```python
from build123d import *

# Parameters (mm, degrees)
SKETCH1_W            = 40
SKETCH1_H            = 40
BOSS_EXTRUDE3_DEPTH  = 2
BOSS_EXTRUDE4_DEPTH  = 6
BOSS_EXTRUDE5_DEPTH  = 2
BOSS_EXTRUDE6_START  = -6
BOSS_EXTRUDE6_DEPTH  = 6
BOSS_EXTRUDE7_DEPTH  = 2
SKETCH7_R            = 1
CUT_EXTRUDE1_DEPTH   = 5
CUT_EXTRUDE2_DEPTH   = 34
BOSS_EXTRUDE8_DEPTH  = 8
BOSS_EXTRUDE9_DEPTH  = 40
SKETCH11_W           = 40
SKETCH11_H           = 40
BOSS_EXTRUDE10_DEPTH = 2
SKETCH13_R           = 1
CUT_EXTRUDE3_DEPTH   = 5
CIRPATTERN1_COUNT    = 4


with BuildPart() as part:
    # Sketch1 → Boss-Extrude3 (new body)
    with BuildSketch(Plane(origin=(0, 0, 0), x_dir=(1, 0, 0), z_dir=(0, 1, 0))):
        Rectangle(SKETCH1_W, SKETCH1_H)
    extrude(amount=BOSS_EXTRUDE3_DEPTH)

    # Sketch5 → Boss-Extrude4 (add)
    with BuildSketch(Plane(origin=(0, 2, 0), x_dir=(1, 0, 0), z_dir=(0, 1, 0))):
        Polygon((18, -10.5), (-18, -10.5), (-18, -12.5), (20, -12.5), (20, 12.5), (-18, 12.5), (-18, 10.5), (18, 10.5), align=None)
    extrude(amount=BOSS_EXTRUDE4_DEPTH)

    # Sketch6 → Boss-Extrude5 (add)
    with BuildSketch(Plane(origin=(0, 8, 0), x_dir=(1, 0, 0), z_dir=(0, 1, 0))):
        with BuildLine():
            ThreePointArc((14, -10.5), (12, -9.5), (10, -10.5))
            Line((10, -10.5), (-10, -10.5))
            ThreePointArc((-10, -10.5), (-12, -9.5), (-14, -10.5))
            Line((-14, -10.5), (-18, -10.5))
            Line((-18, -10.5), (-18, -12.5))
            Line((-18, -12.5), (-14.449489743, -12.5))
            ThreePointArc((-14.449489743, -12.5), (-12, -14.5), (-9.550510257, -12.5))
            Line((-9.550510257, -12.5), (9.550510257, -12.5))
            ThreePointArc((9.550510257, -12.5), (12, -14.5), (14.449489743, -12.5))
            Line((14.449489743, -12.5), (20, -12.5))
            Line((20, -12.5), (20, 12.5))
            Line((20, 12.5), (14.449489743, 12.5))
            ThreePointArc((14.449489743, 12.5), (12, 14.5), (9.550510257, 12.5))
            Line((9.550510257, 12.5), (-9.550510257, 12.5))
            ThreePointArc((-9.550510257, 12.5), (-12, 14.5), (-14.449489743, 12.5))
            Line((-14.449489743, 12.5), (-18, 12.5))
            Line((-18, 12.5), (-18, 10.5))
            Line((-18, 10.5), (-14, 10.5))
            ThreePointArc((-14, 10.5), (-12, 9.5), (-10, 10.5))
            Line((-10, 10.5), (10, 10.5))
            ThreePointArc((10, 10.5), (12, 9.5), (14, 10.5))
            Line((14, 10.5), (18, 10.5))
            Line((18, 10.5), (18, -10.5))
            Line((18, -10.5), (14, -10.5))
        make_face()
    extrude(amount=BOSS_EXTRUDE5_DEPTH)

    # Sketch6<3> → Boss-Extrude6 (add)
    with BuildSketch(Plane(origin=(0, 8, 0), x_dir=(1, 0, 0), z_dir=(0, 1, 0)).offset(BOSS_EXTRUDE6_START)):
        with BuildLine():
            ThreePointArc((-9.550510257, 12.5), (-12, 14.5), (-14.449489743, 12.5))
            Line((-14.449489743, 12.5), (-9.550510257, 12.5))
        make_face()
        with BuildLine():
            ThreePointArc((14.449489743, 12.5), (12, 14.5), (9.550510257, 12.5))
            Line((9.550510257, 12.5), (14.449489743, 12.5))
        make_face()
        with BuildLine():
            Line((-9.550510257, -12.5), (-14.449489743, -12.5))
            ThreePointArc((-14.449489743, -12.5), (-12, -14.5), (-9.550510257, -12.5))
        make_face()
        with BuildLine():
            ThreePointArc((9.550510257, -12.5), (12, -14.5), (14.449489743, -12.5))
            Line((14.449489743, -12.5), (9.550510257, -12.5))
        make_face()
    extrude(amount=BOSS_EXTRUDE6_DEPTH)

    # Sketch6<4> → Boss-Extrude7 (add)
    with BuildSketch(Plane(origin=(0, 8, 0), x_dir=(1, 0, 0), z_dir=(0, 1, 0))):
        with BuildLine():
            Line((-15.5, -8), (-18, -8))
            Line((-18, -8), (-18, -10.5))
            Line((-18, -10.5), (-14, -10.5))
            ThreePointArc((-14, -10.5), (-13.118033989, -9.763932023), (-12, -9.5))
            Line((-12, -9.5), (-12, -8))
            Line((-12, -8), (-15.5, -8))
        make_face()
        with BuildLine():
            Line((12, -8), (-12, -8))
            Line((-12, -8), (-12, -9.5))
            ThreePointArc((-12, -9.5), (-10.881966011, -9.763932023), (-10, -10.5))
            Line((-10, -10.5), (10, -10.5))
            ThreePointArc((10, -10.5), (10.881966011, -9.763932023), (12, -9.5))
            Line((12, -9.5), (12, -8))
        make_face()
        with BuildLine():
            Line((12, 9.5), (12, 8))
            Line((12, 8), (15.5, 8))
            Line((15.5, 8), (15.5, -8))
            Line((15.5, -8), (12, -8))
            Line((12, -8), (12, -9.5))
            ThreePointArc((12, -9.5), (13.118033989, -9.763932023), (14, -10.5))
            Line((14, -10.5), (18, -10.5))
            Line((18, -10.5), (18, 10.5))
            Line((18, 10.5), (14, 10.5))
            ThreePointArc((14, 10.5), (13.118033989, 9.763932023), (12, 9.5))
        make_face()
        with BuildLine():
            ThreePointArc((-10, 10.5), (-10.881966011, 9.763932023), (-12, 9.5))
            Line((-12, 9.5), (-12, 8))
            Line((-12, 8), (12, 8))
            Line((12, 8), (12, 9.5))
            ThreePointArc((12, 9.5), (10.881966011, 9.763932023), (10, 10.5))
            Line((10, 10.5), (-10, 10.5))
        make_face()
        with BuildLine():
            Line((-14, 10.5), (-18, 10.5))
            Line((-18, 10.5), (-18, 8))
            Line((-18, 8), (-15.5, 8))
            Line((-15.5, 8), (-12, 8))
            Line((-12, 8), (-12, 9.5))
            ThreePointArc((-12, 9.5), (-13.118033989, 9.763932023), (-14, 10.5))
        make_face()
    extrude(amount=BOSS_EXTRUDE7_DEPTH)

    # Sketch7 → Cut-Extrude1 (cut)
    with BuildSketch(Plane(origin=(0, 10, 0), x_dir=(1, 0, 0), z_dir=(0, 1, 0))):
        with Locations(Location((-12, 12, 0), (0, 0, 270))):
            Circle(SKETCH7_R)
        with Locations(Location((12, 12, 0), (0, 0, 270))):
            Circle(SKETCH7_R)
        with Locations(Location((12, -12, 0), (0, 0, 270))):
            Circle(SKETCH7_R)
        with Locations(Location((-12, -12, 0), (0, 0, 270))):
            Circle(SKETCH7_R)
    extrude(amount=-CUT_EXTRUDE1_DEPTH, mode=Mode.SUBTRACT)

    # Sketch8 → Cut-Extrude2 (cut)
    with BuildSketch(Plane.XY.offset(12.5)):
        with BuildLine():
            ThreePointArc((-8.550510257, 8), (-8.257617038, 8.707106781), (-7.550510257, 9))
            Line((-7.550510257, 9), (7.550510257, 9))
            ThreePointArc((7.550510257, 9), (8.257617038, 8.707106781), (8.550510257, 8))
            Line((8.550510257, 8), (8.550510257, 4))
            ThreePointArc((8.550510257, 4), (8.257617038, 3.292893219), (7.550510257, 3))
            Line((7.550510257, 3), (-7.550510257, 3))
            ThreePointArc((-7.550510257, 3), (-8.257617038, 3.292893219), (-8.550510257, 4))
            Line((-8.550510257, 4), (-8.550510257, 8))
        make_face()
    extrude(amount=-CUT_EXTRUDE2_DEPTH, mode=Mode.SUBTRACT)

    # Sketch9 → Boss-Extrude8 (add)
    with BuildSketch(Plane(origin=(0, 2, 0), x_dir=(1, 0, 0), z_dir=(0, 1, 0))):
        Polygon((-20, 20), (-20, 17.5), (-17.5, 17.5), (17.5, 17.5), (20, 17.5), (20, 20), align=None)
        Polygon((-17.5, -17.5), (-20, -17.5), (-20, -20), (20, -20), (20, -17.5), (17.5, -17.5), align=None)
    extrude(amount=BOSS_EXTRUDE8_DEPTH)

    # Sketch10 → Boss-Extrude9 (add)
    with BuildSketch(Plane.ZY.offset(20)):
        with BuildLine():
            Line((-17.5, 2), (-15.5, 2))
            ThreePointArc((-15.5, 2), (-16.914213562, 2.585786438), (-17.5, 4))
            Line((-17.5, 4), (-17.5, 2))
        make_face()
        with BuildLine():
            ThreePointArc((17.5, 4), (16.914213562, 2.585786438), (15.5, 2))
            Line((15.5, 2), (17.5, 2))
            Line((17.5, 2), (17.5, 4))
        make_face()
    extrude(amount=-BOSS_EXTRUDE9_DEPTH)

    # Sketch11 → Boss-Extrude10 (add)
    with BuildSketch(Plane.XZ):
        Rectangle(SKETCH11_W, SKETCH11_H)
    extrude(amount=BOSS_EXTRUDE10_DEPTH)

    # Sketch13 → Cut-Extrude3 (cut)
    with BuildSketch(Plane(origin=(20, 0, 0), x_dir=(0, 0, -1), z_dir=(1, 0, 0))):
        with Locations((-10, 0)):
            Circle(SKETCH13_R)
        with Locations(Location((10, 0, 0), (0, 0, 180))):
            Circle(SKETCH13_R)
    cut_extrude3 = extrude(amount=-CUT_EXTRUDE3_DEPTH, mode=Mode.SUBTRACT)

    # CirPattern1: Cut-Extrude3 ×4 about axis
    cirpattern1_axis = Axis((0, 0, 0), (0, 1, 0))
    for i in range(1, CIRPATTERN1_COUNT):
        add(cut_extrude3.rotate(cirpattern1_axis, i * 360 / CIRPATTERN1_COUNT), mode=Mode.SUBTRACT)


solid = part.part
```
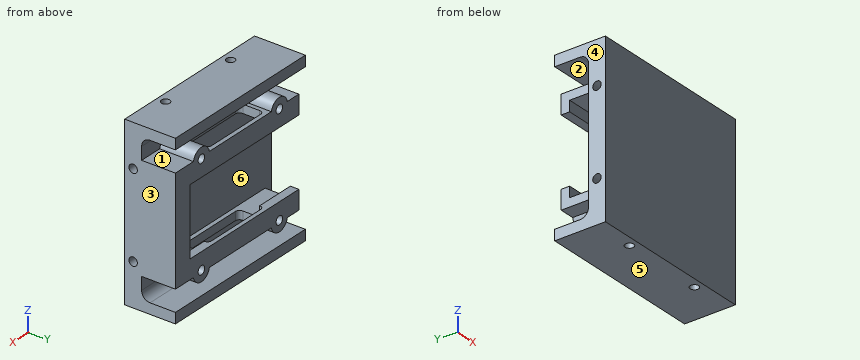
Here's how the part is built. I have some questions about the finished solid (model axes, mm). Face numbers are marked on the shaded views. A direction names the side the tool comes from. Coordinates: 2 decimals unless noted, no trailing zeros. Loops run counter-clockwise (first coordinate to the right, second up) from the corner with the lowest first, then second, coordinate; pieces in that order, holes last. Notation, with made-up numbers: M 51,-22.5 L 75,-22.5 A20 cw 75,8.5 Z; hole C 84,69 d6. An arc over 180 degrees is marked long. One line per item, written item: value.
1. Imagine slicing it at B-B (z = 12). List the corners of the cut face in (x, y) for me.
Geometry says:
outline: M -20,-2 L 20,-2 L 20,10 L 13,10 L 13,5 L 11,5 L 11,10 L -11,10 L -11,5 L -13,5 L -13,10 L -18,10 L -18,2 L -20,2 Z; hole M -8.55,4 A1 ccw -7.55,3 L 7.55,3 A1 ccw 8.55,4 L 8.55,8 A1 ccw 7.55,9 L -7.55,9 A1 ccw -8.55,8 Z
2. Imagine slicing it at C-C (z = 6). List the corners of the cut face in (x, y) for me.
Geometry says:
outline: M -20,-2 L 20,-2 L 20,10 L 15.5,10 L 15.5,8 L 18,8 L 18,2 L -20,2 Z
3. Please list where these lines run through material, in increasing order: probe 1 along X at (y, z) = (6.05, -12); probe 2 along Z at (x, y) = (-8, 5.25); probe 3 along Y at (x, z) = (11, -10).
Geometry says:
probe 1: x = -18 to -13, -11 to -8.55, 8.55 to 11, 13 to 20
probe 2: z = -20 to -17.5, 17.5 to 20
probe 3: y = -2 to 2, 8 to 10
4. Imagine slicing it at D-D (y = 2.5). List the corners of the cut face in (x, z) for me, and give its area (3 significant figures).
Geometry says:
outline: M -20,-20 L 20,-20 L 20,-16.82 L -20,-16.82 Z; M -20,16.82 L 20,16.82 L 20,20 L -20,20 Z; M -18,-12.5 L -14.45,-12.5 A2.5 ccw -9.55,-12.5 L 9.55,-12.5 A2.5 ccw 14.45,-12.5 L 20,-12.5 L 20,12.5 L 14.45,12.5 A2.5 ccw 9.55,12.5 L -9.55,12.5 A2.5 ccw -14.45,12.5 L -18,12.5 L -18,10.5 L 18,10.5 L 18,-10.5 L -18,-10.5 Z
area: 478 mm2
5. Imagine slicing it at A-A (x = 7). List the corners of the cut face in (y, z) for me, and give its area (3 significant figures).
Geometry says:
outline: M -2,-20 L 10,-20 L 10,-17.5 L 4,-17.5 A2 cw 2,-15.5 L 2,-12.5 L 3,-12.5 L 3,-10.5 L 2,-10.5 L 2,10.5 L 3,10.5 L 3,12.5 L 2,12.5 L 2,15.5 A2 cw 4,17.5 L 10,17.5 L 10,20 L -2,20 Z; M 9,-12.5 L 10,-12.5 L 10,-8 L 9,-8 Z; M 9,8 L 10,8 L 10,12.5 L 9,12.5 Z
area: 215 mm2
6. Will these pins go through, and if not, where does the flat tip stop? pin 1 Ø2 at (y, z) = (4.5, 9) entering from -X; pin 2 Ø6 at (y, z) = (6, 1) entering from -X; pin 3 Ø1.2 at (y, z) = (0, -10) entering from -X.
Geometry says:
pin 1: stops at x = 18
pin 2: stops at x = 15.5
pin 3: stops at x = -15
7. On a 3-axis mill with a long thin cutter (end or side, diameter ignored), from which of +Z, -Z, +X, -X, +Y, -Y can I reach the whole of each face in a straight line? I mean the marked faces 1, 2 and 3. Say none if no direction works.
Geometry says:
face 1: +X, +Y
face 2: +X, -X, +Y
face 3: +Z, -Z, +X, +Y, -Y
8. Thinking about a two-plate mould opening in Z: for the marked faces 4, 5 and 6, which applies, +Z half, -Z half, draft (parallel to the pull), parting line (faces both ways), or undercut?
Geometry says:
face 4: draft
face 5: -Z half
face 6: undercut
